CAD build for the part. Positions are in the model's coordinates, mm. A direction names the side the tool comes from. Coordinates: 2 decimals unless noted, no trailing zeros. Loops run counter-clockwise (first coordinate to the right, second up) from the corner with the lowest first, then second, coordinate; pieces in that order, holes last. Notation, with made-up numbers: (-0.75, 59.5) -> (19.25, 59.5) arc R12 cw to (19.25, 82.5) -> close; hole circle Ø1 at (53.25, -4.5). An arc over 180 degrees is marked (long way). Write item = value, one per line. Start each with the question number.
(1) Tool access for faces 4 (the face through (-93, 220, 16)), 5 (the face through (-90, 215.728, 7)), 6 (the face through (-90, 217, 13.25)), 7 (the face through (-99, 232.2, 8)): list every direction of +Z, -Z, +X, -X, +Y, -Y with a clear straight run to the whole face (end or side of a thin tool).
(2) Band-saw the part on D-D (z = 7.5). Write the cut outline in (x, y).
(3) Band-saw the part on C-C (y = 228). Write the cut outline in (x, z), and give its area (3 significant figures).
(4) Flat gauge pins, fed straight in: P1, Ø5.5, axis at x = -90, z = 6.5, coming from the -Y side; P2, Ø8, axis at y = 227, z = 10, coming from the +X side; P3, Ø1.8, axis at x = -94.84, z = 13.5, coming from the -Y side; P4, Ø0.9, axis at x = -90.5, y = 234, coming from the +Z side. Where does each tip first touch, or does it go through?
(5) Drill centre lines: line 1 (X direction, y = 216.7, z = 2.2); line 2 (X direction, y = 227.5, z = 12.5); line 3 (Y direction, x = -98.25, z = 14). Where is each one in solid material? Low to high. Write a range as from..to.
(6) Band-saw the part on B-B (x = -97). Write the cut outline in (y, z), and give its area (3 significant figures).
(7) Band-saw the part on A-A (z = 2.2). Write the cut outline in (x, y), and give its area (3 significant figures).
(8) Pull direction Z, two halves, no side cores. Call faces 1 (the face through (-93.846, 233.786, 13.37)), 2 (the face through (-90, 218.728, 7)), 3 (the face through (-87.218, 217.207, 12.965)): +Z half, -Z half, draft (parallel to the pull), parting line (faces both ways), or undercut.
```python
from build123d import *

# Parameters (mm, degrees)
SKETCH2_W           = 14.6
SKETCH2_H           = 32
BOSS_EXTRUDE1_DEPTH = 16
FILLET1_R           = 1
SKETCH3_W           = 11.9
SKETCH3_H           = 24.4
CUT_EXTRUDE1_DEPTH  = 16
SKETCH4_R           = 1
CUT_EXTRUDE2_DEPTH  = 16
SKETCH5_R           = 1
CUT_EXTRUDE3_DEPTH  = 113.555199241
SKETCH6_W           = 5.2
SKETCH6_H           = 13.25
BOSS_EXTRUDE2_DEPTH = 3
SKETCH7_W           = 5.2
SKETCH7_H           = 13.25
BOSS_EXTRUDE3_DEPTH = 3
SKETCH8_R           = 1
CUT_EXTRUDE4_DEPTH  = 33
FILLET2_R           = 1


with BuildPart() as part:
    # Sketch2 → Boss-Extrude1 (new body)
    with BuildSketch(Plane.XY):
        with Locations((-99.41772522, 219.327818509)):
            Rectangle(SKETCH2_W, SKETCH2_H)
    extrude(amount=BOSS_EXTRUDE1_DEPTH)

    # Fillet1
    fillet1_edges = [part.edges().sort_by_distance(p)[0] for p in [
        (-106.71772522, 235.327818509, 8),
        (-92.11772522, 203.327818509, 8),
        (-106.71772522, 203.327818509, 8),
    ]]
    fillet(fillet1_edges, radius=FILLET1_R)

    # Sketch3 → Cut-Extrude1 (cut)
    with BuildSketch(Plane.XY.offset(16)):
        with Locations((-99.26772522, 219.999996948)):
            Rectangle(SKETCH3_W, SKETCH3_H)
    extrude(amount=-CUT_EXTRUDE1_DEPTH, mode=Mode.SUBTRACT)

    # Sketch4 → Cut-Extrude2 (cut)
    with BuildSketch(Plane.XY.offset(16)):
        with Locations((-99.709122305, 233.799996948)):
            Circle(SKETCH4_R)
        with Locations((-99.709122305, 206.199996948)):
            Circle(SKETCH4_R)
    extrude(amount=-CUT_EXTRUDE2_DEPTH, mode=Mode.SUBTRACT)

    # Sketch5 → Cut-Extrude3 (cut, through all)
    with BuildSketch(Plane(origin=(0, 235.327818509, 0), x_dir=(1, 0, 0), z_dir=(0, 1, 0))):
        with Locations(Location((-103.837557169, -5.5, 0), (0, 0, 270))):
            Circle(SKETCH5_R)
        with Locations(Location((-94.837557169, -5.5, 0), (0, 0, 270))):
            Circle(SKETCH5_R)
        with Locations(Location((-94.837557169, -13.5, 0), (0, 0, 270))):
            Circle(SKETCH5_R)
        with Locations(Location((-103.837557169, -13.5, 0), (0, 0, 270))):
            Circle(SKETCH5_R)
    extrude(amount=-CUT_EXTRUDE3_DEPTH, mode=Mode.SUBTRACT)

    # Sketch6 → Boss-Extrude2 (add)
    with BuildSketch(Plane(origin=(0, 235.327818509, 0), x_dir=(1, 0, 0), z_dir=(0, 1, 0))):
        with Locations((-89.51772522, -6.625)):
            Rectangle(SKETCH6_W, SKETCH6_H)
    extrude(amount=-BOSS_EXTRUDE2_DEPTH)

    # Sketch7 → Boss-Extrude3 (add)
    with BuildSketch(Plane(origin=(0, 218.727818509, 0), x_dir=(1, 0, 0), z_dir=(0, 1, 0))):
        with Locations((-89.51772522, -6.625)):
            Rectangle(SKETCH7_W, SKETCH7_H)
    extrude(amount=-BOSS_EXTRUDE3_DEPTH)

    # Sketch8 → Cut-Extrude4 (cut)
    with BuildSketch(Plane(origin=(0, 235.327818509, 0), x_dir=(1, 0, 0), z_dir=(0, 1, 0))):
        with Locations(Location((-88.91772522, -2.2, 0), (0, 0, 270))):
            Circle(SKETCH8_R)
        with Locations(Location((-88.91772522, -10.684490828, 0), (0, 0, 270))):
            Circle(SKETCH8_R)
    extrude(amount=-CUT_EXTRUDE4_DEPTH, mode=Mode.SUBTRACT)

    # Fillet2
    fillet2_edges = [part.edges().sort_by_distance(p)[0] for p in [
        (-86.91772522, 217.227818509, 0),
        (-86.91772522, 217.227818509, 13.25),
        (-86.91772522, 233.827818509, 0),
        (-86.91772522, 233.827818509, 13.25),
    ]]
    fillet(fillet2_edges, radius=FILLET2_R)


solid = part.part
```
Findings below:
q1.face_4 = +Z, +X, -X, +Y, -Y
q1.face_5 = +Z, -Z, +X, -Y
q1.face_6 = +Z, +X, +Y, -Y
q1.face_7 = +Z, -Z
q2.outline = (-106.72, 204.33) arc R1 ccw to (-105.72, 203.33) -> (-93.12, 203.33) arc R1 ccw to (-92.12, 204.33) -> (-92.12, 215.73) -> (-86.92, 215.73) -> (-86.92, 218.73) -> (-92.12, 218.73) -> (-92.12, 232.33) -> (-86.92, 232.33) -> (-86.92, 235.33) -> (-105.72, 235.33) arc R1 ccw to (-106.72, 234.33) -> close; hole (-105.22, 207.8) -> (-93.32, 207.8) -> (-93.32, 232.2) -> (-105.22, 232.2) -> close; hole circle Ø2 at (-99.71, 206.2); hole circle Ø2 at (-99.71, 233.8)
q3.outline = (-106.72, 0) -> (-105.22, 0) -> (-105.22, 16) -> (-106.72, 16) -> close; (-93.32, 0) -> (-92.12, 0) -> (-92.12, 16) -> (-93.32, 16) -> close
q3.area = 43.2 mm²
q4.P1 = 203.4
q4.P2 = -92.12
q4.P3 = through
q4.P4 = 13.25
q5.line_1 = -106.72..-105.22, -93.32..-89.92, -87.92..-86.92
q5.line_2 = -106.72..-105.22, -93.32..-92.12
q5.line_3 = 203.33..207.8, 232.2..235.33
q6.outline = (203.33, 0) -> (207.8, 0) -> (207.8, 16) -> (203.33, 16) -> close; (232.2, 0) -> (235.33, 0) -> (235.33, 16) -> (232.2, 16) -> close
q6.area = 122 mm²
q7.outline = (-106.72, 204.33) arc R1 ccw to (-105.72, 203.33) -> (-93.12, 203.33) arc R1 ccw to (-92.12, 204.33) -> (-92.12, 215.73) -> (-89.92, 215.73) -> (-89.92, 218.73) -> (-92.12, 218.73) -> (-92.12, 232.33) -> (-89.92, 232.33) -> (-89.92, 235.33) -> (-105.72, 235.33) arc R1 ccw to (-106.72, 234.33) -> close; (-87.92, 215.73) -> (-86.92, 215.73) -> (-86.92, 218.73) -> (-87.92, 218.73) -> close; (-87.92, 232.33) -> (-86.92, 232.33) -> (-86.92, 235.33) -> (-87.92, 235.33) -> close; hole (-105.22, 207.8) -> (-93.32, 207.8) -> (-93.32, 232.2) -> (-105.22, 232.2) -> close; hole circle Ø2 at (-99.71, 206.2); hole circle Ø2 at (-99.71, 233.8)
q7.area = 189 mm²
q8.face_1 = undercut
q8.face_2 = draft
q8.face_3 = +Z half
